Autodesk Inventor part; units mm, degrees
ref_plane "YZ Plane" through (0, 0, 0) normal (1, 0, 0) x (0, 1, 0)
ref_plane "XZ Plane" through (0, 0, 0) normal (0, 1, 0) x (-1, 0, 0)
ref_plane "XY Plane" through (0, 0, 0) normal (0, 0, 1) x (1, 0, 0)
sketch "Sketch1" plane through (0, 0, 0) normal (0, 0, 1) x (1, 0, 0)
  arc A0 (-18.9737, -13) -> (22.5323, -4.6147) centre (0, 0) ccw
  circle A1 centre (0, 0) radius 23 construction
  line L0 (-28, 0) -> (-28, -39.6186) construction
  line L1 (-18.9737, -13) -> (-28, -13)
  line L2 (-28, -13) -> (-28, -15.8)
  line L3 (-28, -15.8) -> (-33, -15.8)
  line L4 (-33, -15.8) -> (-33, -25.8)
  line L5 (37, -25.8) -> (37, -15.8)
  line L6 (37, -15.8) -> (32, -15.8)
  line L7 (32, -15.8) -> (32, 17.2)
  line L8 (-33, -25.8) -> (-28, -25.8)
  line L9 (-28, -33) -> (-28, -25.8)
  line L10 (-28, -33) -> (32, -33)
  line L11 (32, -33) -> (32, -25.8)
  line L12 (32, -25.8) -> (37, -25.8)
  line L13 (0, 0) -> (-28, 0) construction
  line L14 (22.5323, -4.6147) -> (27, 17.2)
  line L15 (27, 17.2) -> (32, 17.2)
  dimension "d0" = 46
  dimension "d1" = 15.8
  dimension "d2" = 13
  dimension "d3" = 5
  dimension "d4" = 5
  dimension "d5" = 10
  dimension "d6" = 60
  dimension "d7" = 33
  dimension "d10" = 33
  dimension "d13" = 28
  dimension "d14" = 5
extrude "Extrusion1" add sketch "Sketch1" along normal blind 5
fillet "Fillet1" radius 3 2 edges at (-18.9737, -13, 2.5) (27, 17.2, 2.5)
equation "\"d4\" = d3"
properties part number "104.003.01_Endanschlag_Flasche"
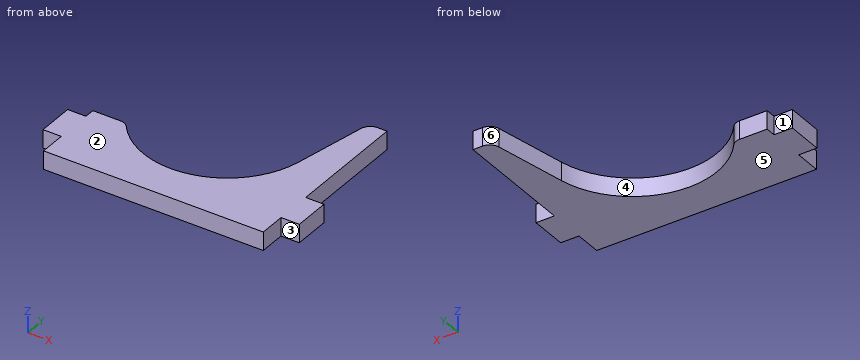
Can you work these out from the model? Positions are in its coordinate system, mm. Face numbers are marked on the shaded views. A direction names the side the tool comes from. Give positions to 0.01 mm unless a question says otherwise; leave off trailing zeros. Loops run counter-clockwise (first coordinate to the right, second up) from the corner with the lowest first, then second, coordinate; pieces in that order, holes last. Notation, with made-up numbers: (43, 40) - (91, 40) arc R17 ccw to (91, 58) - close; hole circle Ø10 at (45, -14.5). An arc over 180 degrees is marked (long way). One line per item, written item: value.
(1) If we section it at B-B, the plane z = 4.1: List the corners of the cut face in (x, y) for me, plus the area to 3 significant figures.
Verdict:
outline: (-33, -25.8) - (-28, -25.8) - (-28, -33) - (32, -33) - (32, -25.8) - (37, -25.8) - (37, -15.8) - (32, -15.8) - (32, 17.2) - (29.45, 17.2) arc R3 ccw to (26.51, 14.8) - (22.53, -4.61) arc R23 cw to (-18.13, -14.15) arc R3 ccw to (-20.49, -13) - (-28, -13) - (-28, -15.8) - (-33, -15.8) - close
area: 1,280 mm^2
(2) If we section it at A-A, the plane y = -20: List the corners of the cut face in (x, z) for me.
Verdict:
outline: (-33, 0) - (-11.36, 0) - (-11.36, 5) - (-33, 5) - close; (11.36, 0) - (37, 0) - (37, 5) - (11.36, 5) - close
(3) I need wall thicknesses on line 1 along X through (y, z) = (-30, 2.3); line 2 along X through (y, z) = (-17.5, 2.45); line 3 along X through (y, z) = (-20, 3.9). Which ranges of each line are inside material? Lowest first, please.
Verdict:
line 1: -28 to 32
line 2: -33 to -14.92, 14.92 to 37
line 3: -33 to -11.36, 11.36 to 37
(4) If we section it at D-D, the plane y = -8: List the corners of the cut face in (x, z) for me, plus the area to 3 significant figures.
Verdict:
outline: (21.56, 0) - (32, 0) - (32, 5) - (21.56, 5) - close
area: 52.2 mm^2
(5) If we mould it in two halves opening along X, with no side actions, what happens to the marked faces 4, 5 and 6? For each: released by +X, released by -X, zero draft, split by the parting line, or undercut.
Verdict:
face 4: undercut
face 5: zero draft
face 6: released by -X
(6) If we section it at C-C, the plane x = -27: List the corners of the cut face in (y, z) for me.
Verdict:
outline: (-33, 0) - (-13, 0) - (-13, 5) - (-33, 5) - close
(7) I'm going to push flat-ended pins straight in: pin 1 (1.5 mm diameter, centred on y = -30.5, z = 1.5, fed in from -X); pin 2 (2.5 mm diameter, centred on x = 34, z = 3.5, fed in from -Y); pin 3 (2.5 mm diameter, centred on x = -30, z = 1.5, fed in from +Y). Where does each tip first touch, or does it pass through?
Verdict:
pin 1: x = -28
pin 2: y = -25.8
pin 3: y = -15.8
(8) On a 3-axis mill with a long thin cutter (end or side, diameter ignored), from which of +Z, -Z, +X, -X, +Y, -Y can I reach the whole of each face in a straight line? I mean the marked faces 1, 2 and 3. Say none if no direction works.
Verdict:
face 1: +Z, -Z, -X, +Y
face 2: +Z, +X, -X, +Y, -Y
face 3: +Z, -Z, +X, -Y
